Autodesk Inventor part; units mm, degrees
ref_plane "YZ Plane" through (0, 0, 0) normal (1, 0, 0) x (0, 1, 0)
ref_plane "XZ Plane" through (0, 0, 0) normal (0, 1, 0) x (-1, 0, 0)
ref_plane "XY Plane" through (0, 0, 0) normal (0, 0, 1) x (1, 0, 0)
sketch "Sketch1" plane through (0, 0, 0) normal (1, 0, 0) x (0, 1, 0)
  line L0 (0, 0) -> (19.05, 0)
  line L1 (19.05, 0) -> (19.05, -127)
  line L2 (19.05, -127) -> (0, -127)
  line L3 (0, -127) -> (0, 0)
  dimension "d0" = 19.05
  dimension "d1" = 127
extrude "Extrusion1" add sketch "Sketch1" along normal blind 6.35
sketch "Sketch2" plane through (6.35, 0, 0) normal (1, 0, 0) x (0, 0, -1)
  circle A0 centre (5.1751, 15.875) radius 1.7526
  circle A1 centre (5.1751, 5.875) radius 1.7526
  line L0 (127, 19.05) -> (0, 19.05)
  circle A2 centre (54.1717, 15.875) radius 1.7526
  circle A3 centre (54.1717, 5.875) radius 1.7526
  point P0 (0, 0)
  dimension "d4" = 3.5052
  dimension "d5" = 3.5052
  dimension "d6" = 10
  dimension "d7" = 3.175
  dimension "d11" = 3.5052
  dimension "d12" = 48.9966
  dimension "d13" = 3.5052
extrude "Extrusion2" cut sketch "Sketch2" against normal through all
sketch "Sketch3" plane through (0, 0, -127) normal (0, -1, 0) x (1, 0, 0)
  line L0 (6.35, 0) -> (6.35, 127)
  line L1 (0, 0) -> (0, 127)
  line L2 (6.35, 127) -> (0, 127)
  line L3 (0, 127) -> (0, 0)
  line L4 (0, 0) -> (6.35, 0)
  line L5 (6.35, 0) -> (6.35, 127)
  point P0 (0, 127)
extrude "Extrusion3" add sketch "Sketch3" along normal blind 50.8
sketch "Sketch4" plane through (0, -50.8, -127) normal (0, -1, 0) x (1, 0, 0)
  line L0 (6.35, 0) -> (6.35, 127)
  line L1 (6.35, 127) -> (-95.25, 127)
  line L2 (-95.25, 127) -> (-95.25, -76.2)
  line L3 (-95.25, -76.2) -> (6.35, -76.2)
  line L4 (6.35, -76.2) -> (6.35, 127)
  point P0 (0, 127)
  point P1 (6.35, 0)
  dimension "d16" = 203.2
  dimension "d17" = 101.6
extrude "Extrusion4" add sketch "Sketch4" along normal blind 12.7
fillet "Fillet1" radius 19.05 1 edges at (0, -50.8, -63.5)
fillet "Fillet2" radius 19.05 2 edges at (-9.525, -50.8, -127) (3.175, -50.8, -127)
sketch "Sketch5" plane through (0, 0, 0) normal (-1, 0, 0) x (0, 0, 1)
  line L0 (-111.3217, 15.6337) -> (-60.5217, 15.6337)
  line L1 (-60.5217, 15.6337) -> (-60.5217, 6.1087)
  line L2 (-60.5217, 6.1087) -> (-111.3217, 6.1087)
  line L3 (-111.3217, 6.1087) -> (-111.3217, 15.6337)
  circle A0 centre (-54.1717, 5.875) radius 1.7526
  circle A1 centre (-54.1717, 15.875) radius 1.7526
  point P0 (0, 0)
  point P1 (-60.5217, 10.8712)
  dimension "d22" = 9.525
  dimension "d23" = 50.8
  dimension "d26" = 5.0038
  dimension "d27" = 6.35
extrude "Extrusion5" add sketch "Sketch5" along normal blind 95.25 contours L0 L1 L2 L3
sketch "Sketch6" plane through (0, 6.1087, -60.5217) normal (0, 0, 1) x (1, 0, 0)
  line L0 (0, 9.525) -> (-95.25, 9.525)
  line L1 (0, 0) -> (-95.25, 0)
  line L2 (-95.25, 9.525) -> (-44.45, 9.525)
  line L3 (-44.45, 9.525) -> (-44.45, 0)
  line L4 (-44.45, 0) -> (-95.25, 0)
  line L5 (-95.25, 0) -> (-95.25, 9.525)
  point P0 (0, -6.1087)
  dimension "d30" = 50.8
extrude "Extrusion6" add sketch "Sketch6" along normal blind 38.1
sketch "Sketch7" plane through (-95.25, 0, 0) normal (-1, 0, 0) x (0, 0, 1)
  line L0 (-22.4217, 15.6337) -> (-22.4217, 6.1087)
  arc A0 (-22.4217, 15.6337) -> (-22.4217, 6.1087) centre (-24.1894, 10.8712) ccw
  line L1 (-22.4217, 15.6337) -> (-22.4217, 6.1087)
  point P0 (0, 0)
  dimension "d33" = 5.08
extrude "Extrusion7" cut sketch "Sketch7" against normal up to surface (50.8 mm away)
fillet "Fillet3" radius 19.05 3 edges at (0, 6.1087, -85.9217) (0, 10.8712, -111.3217) (0, 15.6337, -85.9217)
properties part number "motor plate"
Input: part model. Units: mm. Frame: model coordinates. A direction names the side the tool comes from. Round coordinates to 2 decimals unless told otherwise and drop trailing zeros. Loops run counter-clockwise (first coordinate to the right, second up) from the corner with the lowest first, then second, coordinate; pieces in that order, holes last. Notation, with made-up numbers: M 17.25,62.5 L 61.25,62.5 A27 cw 61.25,97.5 Z; hole C 45,55.25 d7. An arc over 180 degrees is marked long. Answer in a Markdown table with one row per item. Add a question column.
1. Section D-D (x = -22.5). Output: boundary loops of the cut face in (y, z), and give its area (3 significant figures).
2. Mould query, pull axis X, two halves, no side actions, for faces 5 (the face through (-5.104, 16.532, -86.84)), 6 (the face through (-45, -57, -203.2)), 7 (the face through (-17, 10, -60.522)), 8 (the face through (-44.45, 11, -43)). Classes: released by +X, released by -X, zero draft, split by the parting line, or undercut.
3. Section A-A (x = -51.5). Output: boundary loops of the cut face in (y, z), and give its area (3 significant figures).
4. Set-up query: faces 1 (the face through (3, -6, -127)), 2 (the face through (-5.43, 0.38, -85.91)), 3 (the face through (-62, 15.634, -80)), 4 (the face through (-70.21, 10.96, -29.27)). Return all of +Z, -Z, +X, -X, +Y, -Y with unobstructed straight access to the full face (end or side cutting, diameter ignored); none if empty.
5. Ray query, probe 1 along Y at (x, z) = (-55.5, -54); probe 2 along Y at (x, z) = (-53.5, -14); probe 3 along Z at (x, y) = (-38, 15). Return the intervals inside material, ascending.
6. Section B-B (z = -88.5). Output: boundary loops of the cut face in (x, y).
7. Contact query for flat-ended pins moving along their axis: pin 1 (2 mm diameter, centred on y = 15.88, z = -54.17, fed in from +X); pin 2 (16 mm diameter, centred on x = -28.5, y = 3.5, fed in from +Z); pin 3 (1 mm diameter, centred on x = -8, z = -112.5, fed in from +Y). Output: stop coordinate, or through.
8. Section C-C (y = -29.5). Output: boundary loops of the cut face in (x, z).
Values follow:
| question | item | result |
|---|---|---|
| 1 | outline | M -63.5,-203.2 L -50.8,-203.2 L -50.8,0 L -63.5,0 Z; M 6.11,-111.32 L 15.63,-111.32 L 15.63,-60.52 L 6.11,-60.52 Z |
| 1 | area | 3,060 mm^2 |
| 2 | face 5 | released by -X |
| 2 | face 6 | zero draft |
| 2 | face 7 | undercut |
| 2 | face 8 | undercut |
| 3 | outline | M -63.5,-203.2 L -50.8,-203.2 L -50.8,0 L -63.5,0 Z; M 6.11,-111.32 L 15.63,-111.32 L 15.63,-25.96 A5.08 cw 6.11,-25.96 Z |
| 3 | area | 3,370 mm^2 |
| 4 | face 1 | -Z, +X, -X, +Y |
| 4 | face 2 | +Z, -Z, -X |
| 4 | face 3 | +Z, -Z, -X, +Y |
| 4 | face 4 | +Z, -X |
| 5 | probe 1 | -63.5 to -50.8, 6.11 to 15.63 |
| 5 | probe 2 | -63.5 to -50.8 |
| 5 | probe 3 | -111.32 to -60.52 |
| 6 | outline | M -95.25,-63.5 L 6.35,-63.5 L 6.35,19.05 L 0,19.05 A19.05 cw -10.89,15.63 L -95.25,15.63 L -95.25,6.11 L -19.05,6.11 A19.05 cw 0,-12.94 L 0,-31.75 A19.05 cw -19.05,-50.8 L -95.25,-50.8 Z |
| 7 | pin 1 | x = -44.45 |
| 7 | pin 2 | z = -60.52 |
| 7 | pin 3 | y = 15.94 |
| 8 | outline | M 0,-127 L 6.35,-127 L 6.35,0 L 0,0 Z |
